Input: part model. Units: mm. Frame: model coordinates. A direction names the side the tool comes from. Round coordinates to 2 decimals unless told otherwise and drop trailing zeros. Write each loop counter-clockwise with the first axis right and the second up, starting at its lowest first coordinate (ties: lowest second). Pieces come first, ordered by that corner, then holes. Notation, with made-up numbers: (85.25, -29) - (135.25, -29) arc R22 ccw to (135.25, -21) - close; hole circle Ø3 at (88, 43). An arc over 180 degrees is marked (long way). Use one line per item in the form item = value.
```python
from build123d import *

# Parameters (mm, degrees)
SKETCH1_R           = 22.25
BOSS_EXTRUDE1_DEPTH = 2.5
SKETCH2_R           = 2.7
CUT_EXTRUDE1_DEPTH  = 32.565408282
BOSS_EXTRUDE2_START = -7.3
SKETCH3_R           = 11
BOSS_EXTRUDE2_DEPTH = 19
SKETCH4_R           = 2.5
CUT_EXTRUDE2_DEPTH  = 37.757652265


with BuildPart() as part:
    # Sketch1 → Boss-Extrude1 (new body)
    with BuildSketch(Plane(origin=(0, 0, 0), x_dir=(0, 0, -1), z_dir=(1, 0, 0))):
        Circle(SKETCH1_R)
    extrude(amount=BOSS_EXTRUDE1_DEPTH)

    # Sketch2 → Cut-Extrude1 (cut, through all)
    with BuildSketch(Plane(origin=(2.5, 0, 0), x_dir=(0, 0, -1), z_dir=(1, 0, 0))):
        with Locations((17.45, 0)):
            Circle(SKETCH2_R)
        with Locations((-8.725, 15.112143296)):
            Circle(SKETCH2_R)
        with Locations((-8.725, -15.112143296)):
            Circle(SKETCH2_R)
    extrude(amount=-CUT_EXTRUDE1_DEPTH, mode=Mode.SUBTRACT)

    # Sketch3 → Boss-Extrude2 (add)
    with BuildSketch(Plane(origin=(2.5, 0, 0), x_dir=(0, 0, -1), z_dir=(1, 0, 0)).offset(BOSS_EXTRUDE2_START)):
        Circle(SKETCH3_R)
    extrude(amount=BOSS_EXTRUDE2_DEPTH)

    # Sketch4 → Cut-Extrude2 (cut, through all)
    with BuildSketch(Plane.ZY.offset(4.8)):
        Circle(SKETCH4_R)
    extrude(amount=-CUT_EXTRUDE2_DEPTH, mode=Mode.SUBTRACT)


solid = part.part
```
(1) Material intervals for L1, parallel to Y at x = 9, z = 0; L2, parallel to Y at x = 1, z = 0; L3, parallel to X at y = -6, z = -17, sorted ascending.
Derived:
L1 = -11 to -2.5, 2.5 to 11
L2 = -22.25 to -2.5, 2.5 to 22.25
L3 = 0 to 2.5
(2) Cut plane A-A on z = 0. Output: boundary loops of the cut face in (x, y).
Derived:
outline = (-4.8, -11) - (0, -11) - (0, -22.25) - (2.5, -22.25) - (2.5, -11) - (14.2, -11) - (14.2, -2.5) - (-4.8, -2.5) - close; (-4.8, 2.5) - (14.2, 2.5) - (14.2, 11) - (2.5, 11) - (2.5, 22.25) - (0, 22.25) - (0, 11) - (-4.8, 11) - close
(3) Cut plane C-C on x = -2.75. Output: boundary loops of the cut face in (y, z), then the cut area to 3 significant figures.
Derived:
outline = circle Ø22 at (0, 0); hole circle Ø5 at (0, 0)
area = 360 mm^2
(4) First-contact query: pin 1 Ø6 at (x, y) = (0.5, 6) entering from -Z; pin 2 Ø1.5 at (x, z) = (3, -13.5) entering from -Y; pin 3 Ø1.5 at (x, z) = (7.5, -4.5) entering from -Y. Flat tips, straight axial feed; report the tip coordinate or a pass-through.
Derived:
pin_1 = -22.05
pin_2 = -18.1
pin_3 = -10.34
(5) Cut plane D-D on z = -17.45. Output: boundary loops of the cut face in (x, y), then the cut area to 3 significant figures.
Derived:
outline = (0, -13.8) - (2.5, -13.8) - (2.5, -2.7) - (0, -2.7) - close; (0, 2.7) - (2.5, 2.7) - (2.5, 13.8) - (0, 13.8) - close
area = 55.5 mm^2
(6) Cut plane B-B on y = 0. Output: boundary loops of the cut face in (x, z).
Derived:
outline = (-4.8, -11) - (0, -11) - (0, -14.75) - (2.5, -14.75) - (2.5, -11) - (14.2, -11) - (14.2, -2.5) - (-4.8, -2.5) - close; (-4.8, 2.5) - (14.2, 2.5) - (14.2, 11) - (2.5, 11) - (2.5, 22.25) - (0, 22.25) - (0, 11) - (-4.8, 11) - close; (0, -22.25) - (2.5, -22.25) - (2.5, -20.15) - (0, -20.15) - close
(7) Access query for faces 4 (the face through (8.27, -10.74, 2.38)), 5 (the face through (0, -5, 10)), 6 (the face through (1.27, 17.79, 9.08)). Directions: +Z, -Z, +X, -X, +Y, -Y. A direction counts if a zero-diameter tool reaches every point of the face in a straight line with its end or side. Return the directions, or none.
Derived:
face_4 = +X
face_5 = -X
face_6 = +X, -X
(8) Draft query along Y for faces 1 (the face through (-2.43, -10.74, 2.38)), 2 (the face through (14.2, 0, 3)), 3 (the face through (4.57, -2.44, -0.54)). Return one class per face: released by +Y, released by -Y, zero draft, split by the parting line, or undercut.
Derived:
face_1 = split by the parting line
face_2 = zero draft
face_3 = undercut
